The listing builds one solid part. Answer for the finished solid, in the listing's coordinates (mm). Face numbers are marked on the shaded views. Give positions to 0.01 mm unless a question says otherwise; leave off trailing zeros. Order: outer loops, then holes, each group sorted by start corner. A loop starts at its lowest first (then second) coordinate and runs counter-clockwise, first axis right, second up. Notation, with made-up numbers: (-10.75, 77) - (-4.75, 77) arc R15 cw to (-4.75, 106) - close; hole circle Ø1 at (50, 24.5). An arc over 180 degrees is marked (long way). Answer as a JSON object with one key per item and string values. Group by question number.
Q1. A cutting plane is placed at D-D, the plane z = 3.75. Give the vertices of the cut face in (x, y).
Q2. A cutting plane is placed at A-A, the plane z = -2.5. Give the vertices of the cut face in (x, y).
Q3. The mould has two halves that part along Y. Classify the marked faces 1, 2 and 3: released by +Y, released by -Y, zero draft, split by the parting line, or undercut.
Q4. Consider line 1 (Y direction, x = -86, z = -4); line 2 (X direction, y = 50, z = -1.25); line 3 (Z direction, x = -42.5, y = -25.5). Determine where each line is inside the solid, lowest interval first.
Q5. Given pin 1 (4 mm diameter, centred on x = -54.5, y = 49, fed in from -Z); pin 2 (1.5 mm diameter, centred on y = 32.5, z = -4, fed in from -X); pin 3 (2.5 mm diameter, centred on x = -31, z = -3.5, fed in from +Y), each flat-ended and moving along its own axis, determine where each tip first touches the part or whether it passes through.
from build123d import *

# Parameters (mm, degrees)
F0_W     = 101.6
F0_H     = 101.6
F0_W_2   = 96.52
F0_H_2   = 96.52
F1_DEPTH = 5.08
F2_R     = 5.07999
F3_DEPTH = 5.08
F4_W     = 90.17
F4_H     = 90.17
F5_DEPTH = 7.62


# Not quite as in the source:
# - a fillet or chamfer is up to 0.001 mm smaller than in the source, because OpenCascade refuses the exact size


with BuildPart() as f1:
    # F0 (on Top) → F1 (new body)
    with BuildSketch(Plane.XY):
        with Locations((-46.2021417916, 16.1945652217)):
            Rectangle(F0_W, F0_H)
        with Locations((-46.2021417916, 16.1945652217)):
            Rectangle(F0_W_2, F0_H_2, mode=Mode.SUBTRACT)
        with Locations((-46.2021417916, 16.1945652217)):
            Rectangle(F0_W_2, F0_H_2)
    extrude(amount=F1_DEPTH)

    # F2 (radius 5.08 in the source; OpenCascade refuses exactly that, so slightly less here)
    f2_edges = [f1.edges().sort_by_distance(p)[0] for p in [
        (-97.002142, 16.194565, 5.08),
        (-46.202142, -34.605435, 5.08),
        (4.597858, 16.194565, 5.08),
        (-46.202142, 66.994565, 5.08),
    ]]
    fillet(f2_edges, radius=F2_R)

    # F0 (on Top) → F3 (join)
    with BuildSketch(Plane.XY):
        with Locations((-46.2021417916, 16.1945652217)):
            Rectangle(F0_W_2, F0_H_2)
    extrude(amount=-F3_DEPTH)

    # F4 (on face) → F5 (cut)
    with BuildSketch(Plane(origin=(0, 0, -5.08), x_dir=(1, 0, 0), z_dir=(0, 0, -1))):
        with Locations((-46.2021417916, -16.1945652217)):
            Rectangle(F4_W, F4_H)
    extrude(amount=-F5_DEPTH, mode=Mode.SUBTRACT)


solid = f1.part
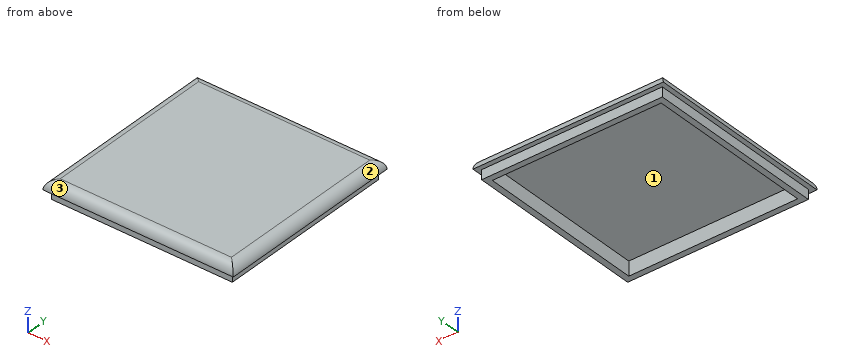
Reply:
{
 "1": {"outline": "(-95.35, -32.95) - (2.94, -32.95) - (2.94, 65.34) - (-95.35, 65.34) - close"},
 "2": {"outline": "(-94.46, -32.07) - (2.06, -32.07) - (2.06, 64.45) - (-94.46, 64.45) - close; hole (-91.29, -28.89) - (-1.12, -28.89) - (-1.12, 61.28) - (-91.29, 61.28) - close"},
 "3": {"face 1": "undercut", "face 2": "zero draft", "face 3": "released by -Y"},
 "4": {"line 1": "y = -32.07 to -28.89, 61.28 to 64.45", "line 2": "x = -94.46 to -91.29, -1.12 to 2.06", "line 3": "z = 2.54 to 5.08"},
 "5": {"pin 1": "stops at z = 2.54", "pin 2": "stops at x = -94.46", "pin 3": "stops at y = 64.45"}
}
